Can you work these out from the model? Positions are in its coordinate system, mm. Face numbers are marked on the shaded views. A direction names the side the tool comes from. Coordinates: 2 decimals unless noted, no trailing zeros. Loops run counter-clockwise (first coordinate to the right, second up) from the corner with the lowest first, then second, coordinate; pieces in that order, holes last.
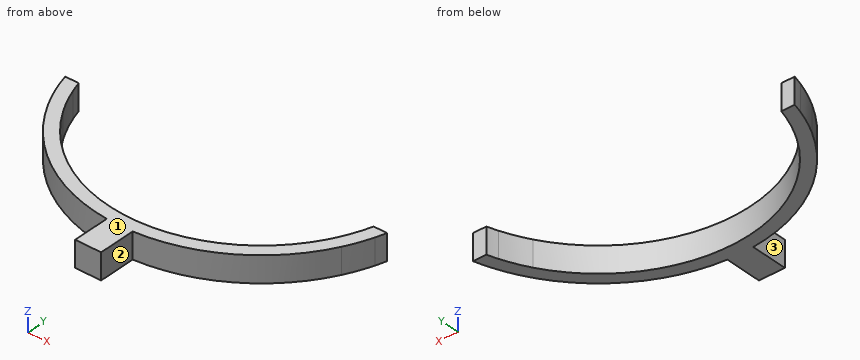
Autodesk Inventor part; units mm, degrees
ref_plane "YZ Plane" through (0, 0, 0) normal (1, 0, 0) x (0, 1, 0)
ref_plane "XZ Plane" through (0, 0, 0) normal (0, 1, 0) x (-1, 0, 0)
ref_plane "XY Plane" through (0, 0, 0) normal (0, 0, 1) x (1, 0, 0)
sketch "Sketch1" plane through (0, 0, 0) normal (0, 0, 1) x (1, 0, 0)
  arc A0 (-25.4018, -15) -> (25.4018, -15) centre (0, 0) ccw
  line L0 (2.5, -32) -> (2.5, -39)
  line L1 (2.5, -39) -> (-2.5, -39)
  line L2 (-2.5, -39) -> (-2.5, -32)
  line L3 (-2.5, -32) -> (-2.5, -31.9022)
  line L4 (2.5, -32) -> (2.5, -31.9022)
  arc A1 (-28.2666, -15) -> (-2.5, -31.9022) centre (0, 0) ccw
  arc A2 (2.5, -31.9022) -> (28.2666, -15) centre (0, 0) ccw
  arc A3 (-27.7534, -10) -> (27.7534, -10) centre (0, 0) ccw
  arc A4 (-30.3974, -10) -> (-2.5, -31.9022) centre (0, 0) ccw
  arc A5 (2.5, -31.9022) -> (30.3974, -10) centre (0, 0) ccw
  arc A6 (-28.3945, -8) -> (28.3945, -8) centre (0, 0) ccw
  line L5 (-28.3945, -8) -> (-30.9839, -8)
  line L6 (28.3945, -8) -> (30.9839, -8)
  arc A7 (-30.9839, -8) -> (-2.5, -31.9022) centre (0, 0) ccw
  arc A8 (2.5, -31.9022) -> (30.9839, -8) centre (0, 0) ccw
  point P0 (25.4018, -15)
  point P1 (-28.2666, -15)
  point P2 (27.7534, -10)
  point P3 (-30.3974, -10)
  dimension "d43" = 5
  dimension "d64" = 7
extrude "Extrusion7" add sketch "Sketch1" along normal blind 5
properties part number "Clip_TestFitV1"
(1) I want a section at D-D on x = 8. Write out the boundary of the cut face in (y, z).
Check values:
outline: (-30.98, 0) - (-28.39, 0) - (-28.39, 5) - (-30.98, 5) - close
(2) I want a section at B-B on z = 1.1. Write out the boundary of the cut face in (x, y).
Check values:
outline: (-30.98, -8) arc R32 ccw to (-30.4, -10) arc R32 ccw to (-28.27, -15) arc R32 ccw to (-2.5, -31.9) - (-2.5, -39) - (2.5, -39) - (2.5, -31.9) arc R32 ccw to (28.27, -15) arc R32 ccw to (30.4, -10) arc R32 ccw to (30.98, -8) - (28.39, -8) arc R29.5 cw to (-25.4, -15) arc R29.5 cw to (-27.75, -10) arc R29.5 cw to (-28.39, -8) - close
(3) I want a section at C-C on y = -27.5. Write out the boundary of the cut face in (x, z), then the cut area to 3 significant figures.
Check values:
outline: (-16.36, 0) - (-10.68, 0) - (-10.68, 5) - (-16.36, 5) - close; (10.68, 0) - (16.36, 0) - (16.36, 5) - (10.68, 5) - close
area: 56.9 mm2
(4) Which directions (+Z, -Z, +X, -X, +Y, -Y) give clear straight access to the entire face, cutting with the end or side of a thin tool? Please do the marked faces 1, 2 and 3.
Check values:
face 1: +Z, +X, -X, +Y, -Y
face 2: +Z, -Z, +X, -Y
face 3: +Z, -Z, -X, -Y
(5) I'm going to push flat-ended pins straight in: pin 1 (1 mm diameter, centred on x = -23, z = 1.5, fed in from +Y); pin 2 (2.5 mm diameter, centred on y = -34.5, z = 3, fed in from -X); pin 3 (1.5 mm diameter, centred on y = -36.5, z = 1.5, fed in from +X). Where does each tip first touch, or does it pass through?
Check values:
pin 1: stops at y = -17.83
pin 2: stops at x = -2.5
pin 3: stops at x = 2.5
(6) I want a section at A-A on y = -11. Write out the boundary of the cut face in (x, z).
Check values:
outline: (-30.05, 0) - (-27.37, 0) - (-27.37, 5) - (-30.05, 5) - close; (27.37, 0) - (30.05, 0) - (30.05, 5) - (27.37, 5) - close
(7) If I drill on probe 1 along X at (y, z) = (-32, 3.5); probe 2 along X at (y, z) = (-27, 3.7); probe 3 along X at (y, z) = (-22, 1), over which ranges is the centre line in solid material (lowest first)?
Check values:
probe 1: x = -2.5 to 2.5
probe 2: x = -17.18 to -11.88, 11.88 to 17.18
probe 3: x = -23.24 to -19.65, 19.65 to 23.24
